Part print with two shaded views. Sizes in mm from the minimum x, y, z corner. Coordinates: 2 decimals unless noted, no trailing zeros. Write each loop counter-clockwise with the first axis right and the second up, starting at its lowest first coordinate (ties: lowest second). Pieces come first, ordered by that corner, then holes.
Q1. Pull direction X, two halves, no side cores. Call the marked faces 1, 2 and 3: released by +X, released by -X, zero draft, split by the parting line, or undercut.
Q2. Band-saw the part on D-D, the plane x = 5. Write the cut outline in (y, z).
Q3. Band-saw the part on A-A, the plane z = 5. Write the cut outline in (x, y), plus the area to 3 significant figures.
Q4. Drill centre lines: probe 1 along Y at (x, z) = (3.25, 6.25); probe 2 along X at (y, z) = (25, 5.5). Where is each one in solid material? Low to high.
Q5. Band-saw the part on B-B, the plane y = 25. Write the cut outline in (x, z).
Q6. Band-saw the part on C-C, the plane y = 15. Write the cut outline in (x, z), plus the area to 3 significant figures.
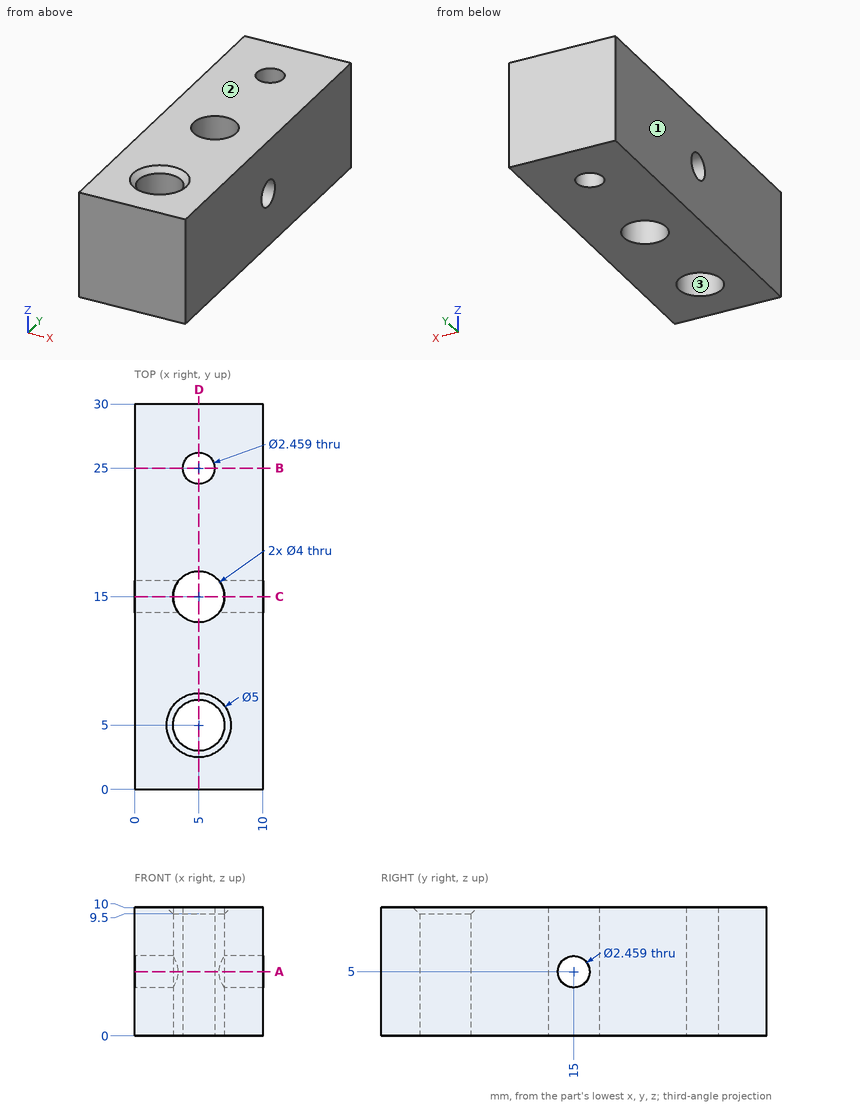
Answer sheet:
1. face 1: released by -X
1. face 2: zero draft
1. face 3: undercut
2. outline: (0, 0) - (3, 0) - (3, 9.5) - (2.5, 10) - (0, 10) - close; (7, 0) - (13, 0) - (13, 10) - (7.5, 10) - (7, 9.5) - close; (17, 0) - (23.77, 0) - (23.77, 10) - (17, 10) - close; (26.23, 0) - (30, 0) - (30, 10) - (26.23, 10) - close
3. outline: (0, 0) - (10, 0) - (10, 13.77) - (6.58, 13.77) arc R2 cw to (3.42, 13.77) - (0, 13.77) - close; (0, 16.23) - (3.42, 16.23) arc R2 cw to (6.58, 16.23) - (10, 16.23) - (10, 30) - (0, 30) - close; hole circle Ø4 at (5, 5); hole circle Ø2.46 at (5, 25)
3. area: 255 mm2
4. probe 1: y = 0 to 4.03, 5.97 to 14.03, 15.97 to 30
4. probe 2: x = 0 to 3.77, 6.23 to 10
5. outline: (0, 0) - (3.77, 0) - (3.77, 10) - (0, 10) - close; (6.23, 0) - (10, 0) - (10, 10) - (6.23, 10) - close
6. outline: (0, 0) - (3, 0) - (3, 3.77) - (0, 3.77) - close; (0, 6.23) - (3, 6.23) - (3, 10) - (0, 10) - close; (7, 0) - (10, 0) - (10, 3.77) - (7, 3.77) - close; (7, 6.23) - (10, 6.23) - (10, 10) - (7, 10) - close
6. area: 45.2 mm2
